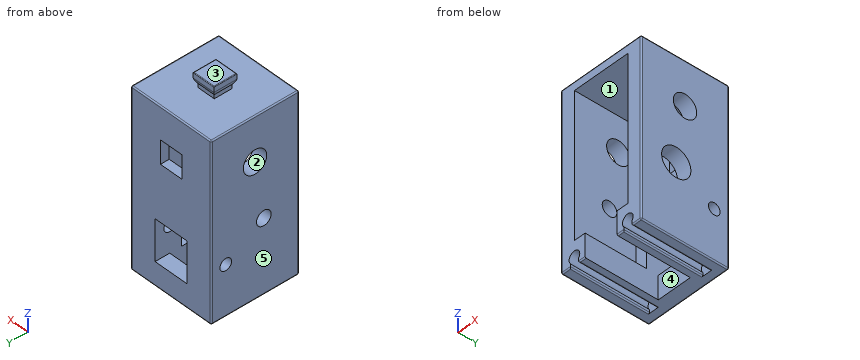
from build123d import *

# Parameters (mm, degrees)
SKETCH_1_W           = 15
SKETCH_1_H           = 15
EXTRUDE_1_DEPTH      = 30
SKETCH_2_W           = 3
SKETCH_2_H           = 3
EXTRUDE_2_DEPTH      = 1
EXTRUDE_3_DEPTH      = 1
EXTRUDE_3_DEPTH_BACK = 4
CUT_EXTRUDE_1_REACH  = 36.847
FILLET_1_R           = 0.1
CUT_EXTRUDE_2_DEPTH  = 13.5
SKETCH_6_W           = 10
SKETCH_6_H           = 8.5
EXTRUDE_4_DEPTH      = 3
SKETCH_7_W           = 6
SKETCH_7_H           = 4
EXTRUDE_5_DEPTH      = 1
SKETCH_8_W           = 6
SKETCH_8_H           = 7
CUT_EXTRUDE_3_DEPTH  = 33.657311586
CUT_EXTRUDE_4_DEPTH  = 13.5
CUT_EXTRUDE_5_REACH  = 36.369
SKETCH_11_W          = 4
SKETCH_11_H          = 4
CUT_EXTRUDE_6_REACH  = 38.742
SKETCH_12_R          = 2.5
SKETCH_12_R_2        = 2
SKETCH_12_R_3        = 1
CUT_EXTRUDE_7_REACH  = 37.795
SKETCH_14_R          = 2
SKETCH_14_R_2        = 1
SKETCH_14_R_3        = 1.25
FILLET_2_R           = 0.2


with BuildPart() as part:
    # 草图1 → 凸台-拉伸1 (new body)
    with BuildSketch(Plane.XY):
        with Locations((0, 7.5)):
            Rectangle(SKETCH_1_W, SKETCH_1_H)
    extrude(amount=-EXTRUDE_1_DEPTH)

    # 草图2 → 凸台-拉伸2 (add)
    with BuildSketch(Plane.XY):
        with Locations((0, 7.5)):
            Rectangle(SKETCH_2_W, SKETCH_2_H)
    extrude(amount=EXTRUDE_2_DEPTH)

    # 草图3 → 凸台-拉伸3 (add, two sides: drawn at the far end of the back side and taken through both)
    with BuildSketch(Plane.XZ.offset(-6).offset(-EXTRUDE_3_DEPTH_BACK)):
        with BuildLine():
            Line((-1.95, 2.5), (1.95, 2.5))
            Line((1.95, 2.5), (1.95, 1.555590279))
            ThreePointArc((1.95, 1.555590279), (1.780042303, 1.088161527), (1.5, 0.677124344))
            Line((1.5, 0.677124344), (-1.5, 0.677124344))
            ThreePointArc((-1.5, 0.677124344), (-1.780042303, 1.088161527), (-1.95, 1.555590279))
            Line((-1.95, 1.555590279), (-1.95, 2.5))
        make_face()
    extrude(amount=EXTRUDE_3_DEPTH + EXTRUDE_3_DEPTH_BACK)

    # 草图4 → 切除-拉伸1 (cut, up to next)
    with BuildSketch(Plane.ZY.offset(1.95), mode=Mode.PRIVATE) as cut_extrude_1_sk1:
        with BuildLine():
            Line((2.5, 9.45), (1.555590279, 9.45))
            ThreePointArc((1.555590279, 9.45), (1.088161527, 9.280042303), (0.677124344, 9))
            Line((0.677124344, 9), (0.677124344, 10))
            Line((0.677124344, 10), (2.5, 10))
            Line((2.5, 10), (2.5, 9.45))
        make_face()
    cut_extrude_1_tool1 = extrude(cut_extrude_1_sk1.sketch, amount=-CUT_EXTRUDE_1_REACH, mode=Mode.PRIVATE) & part.part
    # 草图4 → 切除-拉伸1 (cut, up to next)
    with BuildSketch(Plane.ZY.offset(1.95), mode=Mode.PRIVATE) as cut_extrude_1_sk2:
        with BuildLine():
            Line((2.5, 5.55), (1.555590279, 5.55))
            ThreePointArc((1.555590279, 5.55), (1.088161527, 5.719957697), (0.677124344, 6))
            Line((0.677124344, 6), (0.677124344, 5))
            Line((0.677124344, 5), (2.5, 5))
            Line((2.5, 5), (2.5, 5.55))
        make_face()
    cut_extrude_1_tool2 = extrude(cut_extrude_1_sk2.sketch, amount=-CUT_EXTRUDE_1_REACH, mode=Mode.PRIVATE) & part.part
    add(cut_extrude_1_tool1.solids().sort_by_distance((-1.95, 9.669375, 1.500125))[0], mode=Mode.SUBTRACT)
    add(cut_extrude_1_tool2.solids().sort_by_distance((-1.95, 5.330625, 1.500125))[0], mode=Mode.SUBTRACT)

    # 圆角1
    fillet_1_edges = [part.edges().sort_by_distance(p)[0] for p in [
        (1.95, 7.5, 2.5),
        (-1.95, 7.5, 2.5),
        (0, 9.45, 2.5),
        (0, 5.55, 2.5),
    ]]
    fillet(fillet_1_edges, radius=FILLET_1_R)

    # 草图5 → 切除-拉伸2 (cut)
    with BuildSketch(Plane.XZ):
        Polygon((-5, -1.5), (5, -1.5), (5, -26), (3, -26), (3, -30), (-3, -30), (-3, -26), (-5, -26), align=None)
    extrude(amount=-CUT_EXTRUDE_2_DEPTH, mode=Mode.SUBTRACT)

    # 草图6 → 凸台-拉伸4 (add)
    with BuildSketch(Plane.XZ.offset(-13.5)):
        with Locations((0, -21.75)):
            Rectangle(SKETCH_6_W, SKETCH_6_H)
    extrude(amount=EXTRUDE_4_DEPTH)

    # 草图7 → 凸台-拉伸5 (add)
    with BuildSketch(Plane.XZ.offset(-13.5)):
        with Locations((0, -28)):
            Rectangle(SKETCH_7_W, SKETCH_7_H)
    extrude(amount=EXTRUDE_5_DEPTH)

    # 草图8 → 切除-拉伸3 (cut, through all)
    with BuildSketch(Plane.XZ.offset(-10.5)):
        with Locations((0, -22.5)):
            Rectangle(SKETCH_8_W, SKETCH_8_H)
    extrude(amount=-CUT_EXTRUDE_3_DEPTH, mode=Mode.SUBTRACT)

    # 草图10 → 切除-拉伸4 (cut)
    with BuildSketch(Plane.XZ):
        with BuildLine():
            Line((-5.75, -30), (-5.75, -29.361437828))
            ThreePointArc((-5.75, -29.361437828), (-5, -27.7), (-4.25, -29.361437828))
            Line((-4.25, -29.361437828), (-4.25, -30))
            Line((-4.25, -30), (-5.75, -30))
        make_face()
        with BuildLine():
            Line((5.75, -30), (4.25, -30))
            Line((4.25, -30), (4.25, -29.361437828))
            ThreePointArc((4.25, -29.361437828), (5, -27.7), (5.75, -29.361437828))
            Line((5.75, -29.361437828), (5.75, -30))
        make_face()
    extrude(amount=-CUT_EXTRUDE_4_DEPTH, mode=Mode.SUBTRACT)

    # 草图11 → 切除-拉伸5 (cut, up to next)
    with BuildSketch(Plane(origin=(0, 15, 0), x_dir=(-1, 0, 0), z_dir=(0, 1, 0)), mode=Mode.PRIVATE) as cut_extrude_5_sk1:
        with Locations((0, -7.5)):
            Rectangle(SKETCH_11_W, SKETCH_11_H)
    cut_extrude_5_tool1 = extrude(cut_extrude_5_sk1.sketch, amount=-CUT_EXTRUDE_5_REACH, mode=Mode.PRIVATE) & part.part
    add(cut_extrude_5_tool1.solids().sort_by_distance((0, 15, -7.5))[0], mode=Mode.SUBTRACT)

    # 草图12 → 切除-拉伸6 (cut, up to next)
    with BuildSketch(Plane(origin=(7.5, 0, 0), x_dir=(0, 0, -1), z_dir=(1, 0, 0)), mode=Mode.PRIVATE) as cut_extrude_6_sk1:
        with Locations((17.5, 6)):
            Circle(SKETCH_12_R)
    cut_extrude_6_tool1 = extrude(cut_extrude_6_sk1.sketch, amount=-CUT_EXTRUDE_6_REACH, mode=Mode.PRIVATE) & part.part
    # 草图12 → 切除-拉伸6 (cut, up to next)
    with BuildSketch(Plane(origin=(7.5, 0, 0), x_dir=(0, 0, -1), z_dir=(1, 0, 0)), mode=Mode.PRIVATE) as cut_extrude_6_sk2:
        with Locations((7.5, 7.5)):
            Circle(SKETCH_12_R_2)
    cut_extrude_6_tool2 = extrude(cut_extrude_6_sk2.sketch, amount=-CUT_EXTRUDE_6_REACH, mode=Mode.PRIVATE) & part.part
    # 草图12 → 切除-拉伸6 (cut, up to next)
    with BuildSketch(Plane(origin=(7.5, 0, 0), x_dir=(0, 0, -1), z_dir=(1, 0, 0)), mode=Mode.PRIVATE) as cut_extrude_6_sk3:
        with Locations((21.5, 12.5)):
            Circle(SKETCH_12_R_3)
    cut_extrude_6_tool3 = extrude(cut_extrude_6_sk3.sketch, amount=-CUT_EXTRUDE_6_REACH, mode=Mode.PRIVATE) & part.part
    add(cut_extrude_6_tool1.solids().sort_by_distance((7.5, 6, -17.5))[0], mode=Mode.SUBTRACT)
    add(cut_extrude_6_tool2.solids().sort_by_distance((7.5, 7.5, -7.5))[0], mode=Mode.SUBTRACT)
    add(cut_extrude_6_tool3.solids().sort_by_distance((7.5, 12.5, -21.5))[0], mode=Mode.SUBTRACT)

    # 草图14 → 切除-拉伸7 (cut, up to next)
    with BuildSketch(Plane(origin=(-5, 0, 0), x_dir=(0, 0, -1), z_dir=(1, 0, 0)), mode=Mode.PRIVATE) as cut_extrude_7_sk1:
        with Locations((7.5, 7.5)):
            Circle(SKETCH_14_R)
    cut_extrude_7_tool1 = extrude(cut_extrude_7_sk1.sketch, amount=-CUT_EXTRUDE_7_REACH, mode=Mode.PRIVATE) & part.part
    # 草图14 → 切除-拉伸7 (cut, up to next)
    with BuildSketch(Plane(origin=(-5, 0, 0), x_dir=(0, 0, -1), z_dir=(1, 0, 0)), mode=Mode.PRIVATE) as cut_extrude_7_sk2:
        with Locations((21.5, 12.5)):
            Circle(SKETCH_14_R_2)
    cut_extrude_7_tool2 = extrude(cut_extrude_7_sk2.sketch, amount=-CUT_EXTRUDE_7_REACH, mode=Mode.PRIVATE) & part.part
    # 草图14 → 切除-拉伸7 (cut, up to next)
    with BuildSketch(Plane(origin=(-5, 0, 0), x_dir=(0, 0, -1), z_dir=(1, 0, 0)), mode=Mode.PRIVATE) as cut_extrude_7_sk3:
        with Locations((17.5, 6)):
            Circle(SKETCH_14_R_3)
    cut_extrude_7_tool3 = extrude(cut_extrude_7_sk3.sketch, amount=-CUT_EXTRUDE_7_REACH, mode=Mode.PRIVATE) & part.part
    add(cut_extrude_7_tool1.solids().sort_by_distance((-5, 7.5, -7.5))[0], mode=Mode.SUBTRACT)
    add(cut_extrude_7_tool2.solids().sort_by_distance((-5, 12.5, -21.5))[0], mode=Mode.SUBTRACT)
    add(cut_extrude_7_tool3.solids().sort_by_distance((-5, 6, -17.5))[0], mode=Mode.SUBTRACT)

    # 圆角2
    fillet_2_edges = [part.edges().sort_by_distance(p)[0] for p in [
        (7.5, 7.5, -30),
        (0, 15, -30),
        (-3.625, 0, -30),
        (-4.25, 6.75, -30),
        (-5.75, 6.75, -30),
        (6.625, 0, -30),
        (5.75, 6.75, -30),
        (4.25, 6.75, -30),
        (-7.5, 7.5, -30),
        (0, 15, 0),
        (7.5, 7.5, 0),
        (0, 0, 0),
        (-7.5, 7.5, 0),
        (-6.625, 0, -30),
        (-7.5, 15, -15),
        (7.5, 15, -15),
        (7.5, 0, -15),
        (-7.5, 0, -15),
        (3.625, 0, -30),
    ]]
    fillet(fillet_2_edges, radius=FILLET_2_R)


solid = part.part
Input: part model. Units: mm. Frame: model coordinates. Face numbers are marked on the shaded views. A direction names the side the tool comes from. Coordinates: 2 decimals unless noted, no trailing zeros. Order: outer loops, then holes, each group sorted by start corner. A loop starts at its lowest first (then second) coordinate and runs counter-clockwise, first axis right, second up.
1. Draft query along X for the marked faces 3, 4 and 5. Return one class per face: +X half, -X half, draft (parallel to the pull), parting line (faces both ways), or undercut.
Checked values:
face 3: draft
face 4: undercut
face 5: -X half
2. Cut plane B-B, the plane y = 11. Return loops of the section in (x, z).
Checked values:
outline: (-7.5, -29.8) arc R0.2 ccw to (-7.3, -30) - (-5.95, -30) arc R0.2 ccw to (-5.75, -29.8) - (-5.75, -29.36) arc R1 cw (long way) to (-4.25, -29.36) - (-4.25, -29.8) arc R0.2 ccw to (-4.05, -30) - (-3, -30) - (-3, -19) - (3, -19) - (3, -30) - (4.05, -30) arc R0.2 ccw to (4.25, -29.8) - (4.25, -29.36) arc R1 cw (long way) to (5.75, -29.36) - (5.75, -29.8) arc R0.2 ccw to (5.95, -30) - (7.3, -30) arc R0.2 ccw to (7.5, -29.8) - (7.5, -0.2) arc R0.2 ccw to (7.3, 0) - (-7.3, 0) arc R0.2 ccw to (-7.5, -0.2) - close; hole (-5, -17.5) - (5, -17.5) - (5, -1.5) - (-5, -1.5) - close
3. Cut plane D-D, the plane z = -21.5. Return loops of the section in (x, y), plus the area to 3 significant figures.
Checked values:
outline: (-7.5, 0.2) arc R0.2 ccw to (-7.3, 0) - (-5, 0) - (-5, 10.5) - (-3, 10.5) - (-3, 15) - (-7.3, 15) arc R0.2 ccw to (-7.5, 14.8) - (-7.5, 13.5) - (-5, 13.5) - (-5, 11.5) - (-7.5, 11.5) - close; (3, 10.5) - (5, 10.5) - (5, 0) - (7.3, 0) arc R0.2 ccw to (7.5, 0.2) - (7.5, 11.5) - (3, 11.5) - close; (3, 13.5) - (7.5, 13.5) - (7.5, 14.8) arc R0.2 ccw to (7.3, 15) - (3, 15) - close
area: 79.0 mm2
4. Contact query for flat-ended pins moving along their axis: P1, Ø0.7, axis at x = 0.5, z = 2, coming from the -Y side; P2, Ø1.2, axis at x = -5, z = -28.7, coming from the -Y side; P3, Ø2.5, axis at x = 1.5, z = -21, coming from the -Y side; P4, Ø0.9, axis at y = 7, z = 2, coming from the +X side. Output: stop coordinate, or through.
Checked values:
P1: stops at y = 5.55
P2: stops at y = 13.5
P3: passes through
P4: stops at x = 1.95
5. Cut plane A-A, the plane z = -25. Return loops of the section in (x, y).
Checked values:
outline: (-7.5, 0.2) arc R0.2 ccw to (-7.3, 0) - (-5, 0) - (-5, 10.5) - (-3, 10.5) - (-3, 15) - (-7.3, 15) arc R0.2 ccw to (-7.5, 14.8) - close; (3, 10.5) - (5, 10.5) - (5, 0) - (7.3, 0) arc R0.2 ccw to (7.5, 0.2) - (7.5, 14.8) arc R0.2 ccw to (7.3, 15) - (3, 15) - close
6. Ray query, line 1 along X through (y, z) = (7, -28.7); line 2 along X through (y, z) = (5.75, -26.5); line 3 along X through (y, z) = (1.75, -9). Return the intervals inside material, ascending.
Checked values:
line 1: x = -7.5 to -6, -4 to -3, 3 to 4, 6 to 7.5
line 2: x = -7.5 to -3, 3 to 7.5
line 3: x = -7.5 to -5, 5 to 7.5
7. Cut plane C-C, the plane x = -0.25. Count the separate pieces of the cut face and the enclosed holes in it, plus the area to 3 significant figures.
Checked values:
separate pieces: 3
enclosed holes: 0
area: 66.0 mm2
8. Access query for the marked faces 1 and 2. Directions: +Z, -Z, +X, -X, +Y, -Y. A direction counts if a zero-diameter tool reaches every point of the face in a straight line with its end or side. Return the directions, or none.
Checked values:
face 1: -Y
face 2: +X, -X
